from build123d import *

# Parameters (mm, degrees)
F3_D    = 28.575
F4_R    = 9.525
F5_SIZE = 5
F6_SIZE = 5


with BuildPart() as f1:
    # F0 (on Front) → F1 (revolve)
    with BuildSketch(Plane.XZ):
        Polygon((38.89502, 109.5), (38.89502, -31.724), (44.1071, -31.724), (47.308175, -24.18274), (56.298425, -24.18274), (59.4995, -31.724), (76.2, -31.724), (76.2, -24.1802), (134.9375, -24.1802), (134.9375, 34.16106), (71.04126, 34.16106), (55.11292, 91.055568), (55.11292, 97.055568), align=None)
    revolve(axis=Axis((0, 0, 78.919753), (0, 0, 1)))

    # F3 (through all)
    with Locations(Plane.XY.offset(34.16106)):
        with Locations((0, 107.95), (76.332177, 76.332177), (107.95, 0), (76.332177, -76.332177), (0, -107.95), (-76.332177, -76.332177), (-107.95, 0), (-76.332177, 76.332177)):
            Hole(F3_D / 2)

    # F4
    f4_edges = [f1.edges().sort_by_distance(p)[0] for p in [
        (-71.04126, 0, 34.16106),
    ]]
    fillet(f4_edges, radius=F4_R)

    # F5
    f5_edges = [f1.edges().sort_by_distance(p)[0] for p in [
        (-134.9375, 0, -24.1802),
    ]]
    chamfer(f5_edges, length=F5_SIZE)

    # F6
    f6_edges = [f1.edges().sort_by_distance(p)[0] for p in [
        (-134.9375, 0, 34.16106),
    ]]
    chamfer(f6_edges, length=F6_SIZE)


solid = f1.part
The model under review builds one solid part; all positions refer to its coordinate system, in mm. A direction names the side the tool comes from. Coordinates: 2 decimals unless noted, no trailing zeros. Write each loop counter-clockwise with the first axis right and the second up, starting at its lowest first coordinate (ties: lowest second). Pieces come first, ordered by that corner, then holes. Notation, with made-up numbers: M 60,-37.5 L 85,-37.5 A6 cw 85,-26.5 Z; hole C 76,82 d2. An arc over 180 degrees is marked long. Put each result on its own line as item: value.
1) Clearance check with flat-ended pins moving along their axes: pin 1 Ø1.5 at (y, z) = (25.5, 22.5) entering from -X; pin 2 Ø8 at (x, y) = (81.5, -85) entering from +Z; pin 3 Ø8 at (x, y) = (79.5, -45.5) entering from -Z; pin 4 Ø2 at (x, z) = (47.5, 10.5) entering from +Y. State where each tip first meets the part, or that it passes through.
Computed:
pin 1: stops at x = -132.65
pin 2: passes through
pin 3: stops at z = -24.18
pin 4: stops at y = 126.67
2) For faces 5 (the flat face through (-56, -56, -24.18)), 6 (the cylindrical face through (-8.43, -37.97, 37.9)), list the 3-axis set-ups (+Z, -Z, +X, -X, +Y, -Y) from which the entire face can be reached by the end or side of a thin tool; tool diameter is ignored.
Computed:
face 5: -Z
face 6: +Z, -Z
3) Draft analysis for pull direction Y (two halves, no side actions). For faces 1 (the cylindrical face through (69.739, 63.657, 4.582)), 2 (the cylindrical face through (-60.47, -46.367, -27.899)), 3 (the cylindrical face through (68.651, -64.285, 4.582)), 4 (the flat face through (46, -39, -31.724)), state which applies: released by +Y, released by -Y, zero draft, split by the parting line, or undercut.
Computed:
face 1: undercut
face 2: split by the parting line
face 3: undercut
face 4: zero draft
4) Add section C-C on z = 87. Give the boundary of the cut face in (x, y).
Computed:
outline: C 0,0 d112.5; hole C 0,0 d77.79
5) Wall thickness on probe 1 along X at (y, z) = (116, 0.5); probe 2 along X at (y, z) = (-18.5, 84); probe 3 along Y at (x, z) = (-66.5, -1.5): over which ranges is each line inside the solid? List them lowest first. Write a range as [from, to].
Computed:
probe 1: x = [-68.94, -11.8], [11.8, 68.94]
probe 2: x = [-54.01, -34.21], [34.21, 54.01]
probe 3: y = [-117.41, -86.7], [-65.97, 65.97], [86.7, 117.41]
6) Add section D-D on z = 51.5. Give the boundary of the cut face in (x, y), then the cut area to 3 significant figures.
Computed:
outline: C 0,0 d132.37; hole C 0,0 d77.79
area: 9,010 mm2
7) Add section A-A on y = 0. State how many separate pieces and enclosed holes the cut face has, then the cut area to 3 significant figures.
Computed:
separate pieces: 4
enclosed holes: 0
area: 11,400 mm2
